Autodesk Inventor part; units mm, degrees
ref_plane "YZ Plane" through (0, 0, 0) normal (1, 0, 0) x (0, 1, 0)
ref_plane "XZ Plane" through (0, 0, 0) normal (0, 1, 0) x (-1, 0, 0)
ref_plane "XY Plane" through (0, 0, 0) normal (0, 0, 1) x (1, 0, 0)
sketch "Sketch1" plane through (0, 0, 0) normal (0, 1, 0) x (-1, 0, 0)
  line L0 (0, 0) -> (-457.2, 0)
  line L1 (-457.2, 0) -> (-457.2, -457.2)
  line L2 (-457.2, -457.2) -> (0, -457.2)
  line L3 (0, -457.2) -> (0, 0)
  dimension "d0" = 457.2
  dimension "d1" = 457.2
extrude "Extrusion1" add sketch "Sketch1" along normal blind 381
sketch "Sketch2" plane through (0, 381, 0) normal (0, 1, 0) x (1, 0, 0)
  line L0 (0, 0) -> (457.2, 0)
  line L1 (457.2, 0) -> (457.2, 457.2)
  line L2 (457.2, 457.2) -> (0, 457.2)
  line L3 (0, 457.2) -> (0, 0)
  line L4 (12.7, 12.7) -> (444.5, 12.7)
  line L5 (444.5, 12.7) -> (444.5, 444.5)
  line L6 (444.5, 444.5) -> (12.7, 444.5)
  line L7 (12.7, 444.5) -> (12.7, 12.7)
  dimension "d4" = 12.7
extrude "Extrusion2" cut sketch "Sketch2" against normal blind 368.3 contours L7 L6 L5 L4
sketch "Sketch3" plane through (0, 0, 0) normal (0, -1, 0) x (1, 0, 0)
  line L0 (0, 0) -> (457.2, 0)
  line L1 (0, -457.2) -> (0, 0)
  line L2 (457.2, -457.2) -> (0, -457.2)
  line L3 (457.2, 0) -> (457.2, -457.2)
  line L4 (457.2, 0) -> (406.4, 0) construction
  line L5 (0, 0) -> (457.2, 0) construction
  line L6 (406.4, 0) -> (406.4, -76.2) construction
  circle A0 centre (406.4, -76.2) radius 15.875
  line L7 (457.2, 0) -> (457.2, -457.2) construction
  line L8 (457.2, -228.6) -> (0, -228.6) construction
  line L9 (228.6, 0) -> (228.6, -457.2) construction
  circle A1 centre (406.4, -381) radius 15.875
  circle A2 centre (50.8, -381) radius 15.875
  circle A3 centre (50.8, -76.2) radius 15.875
  point P0 (228.6, -228.6)
  dimension "d7" = 50.8
  dimension "d8" = 76.2
  dimension "d9" = 31.75
extrude "Extrusion3" cut sketch "Sketch3" against normal blind 25.4 contours A0 | A1 | A2 | A3
sketch "Sketch5" plane through (0, 12.7, 0) normal (0, 1, 0) x (1, 0, 0)
  circle A0 centre (50.8, 381) radius 15.875
  circle A1 centre (406.4, 76.2) radius 15.875
  circle A2 centre (406.4, 381) radius 15.875
  circle A3 centre (50.8, 76.2) radius 15.875
  line L0 (444.5, 12.7) -> (12.7, 12.7)
  line L1 (444.5, 444.5) -> (444.5, 12.7)
  line L2 (12.7, 444.5) -> (444.5, 444.5)
  line L3 (12.7, 12.7) -> (12.7, 444.5)
  circle A4 centre (50.8, 381) radius 22.225
  circle A5 centre (406.4, 381) radius 22.225
  circle A6 centre (50.8, 76.2) radius 22.225
  circle A7 centre (406.4, 76.2) radius 22.225
  point P0 (0, 0)
  dimension "d19" = 6.35
  dimension "d20" = 6.35
  dimension "d21" = 6.35
  dimension "d22" = 6.35
extrude "Extrusion5" add sketch "Sketch5" along normal blind 12.7 contours A4 | A5 | A6 | A7
properties part number "Attachable top" material "PET Plastic"
CAD build for the part. Positions are in the model's coordinates, mm. A direction names the side the tool comes from. Coordinates: 2 decimals unless noted, no trailing zeros. Order: outer loops, then holes, each group sorted by start corner. A loop starts at its lowest first (then second) coordinate and runs counter-clockwise, first axis right, second up. Notation, with made-up numbers: M 53,-33.5 L 57,-33.5 A22 ccw 57,2.5 Z; hole C 33,58.25 d5. An arc over 180 degrees is marked long. Answer as CSV lines item,"result".
1) Cut at A-A (x = 50.8). List the corners of the cut face in (y, z) (3 decimals).
Verdict:
outline,"M 0,-457.2 L 381,-457.2 L 381,-444.5 L 12.7,-444.5 L 12.7,-403.225 L 25.4,-403.225 L 25.4,-396.875 L 0,-396.875 Z; M 0,-365.125 L 25.4,-365.125 L 25.4,-358.775 L 12.7,-358.775 L 12.7,-98.425 L 25.4,-98.425 L 25.4,-92.075 L 0,-92.075 Z; M 0,-60.325 L 25.4,-60.325 L 25.4,-53.975 L 12.7,-53.975 L 12.7,-12.7 L 381,-12.7 L 381,0 L 0,0 Z"
2) 3-axis set-ups, long thin cutter, end or side, ignore diameter. For faces 1 (the flat face through (457.2, 188, -225)), 2 (the flat face through (232, 199, -444.5)): which of +Z, -Z, +X, -X, +Y, -Y reach the whole face in a straight line?
Verdict:
face 1,"+Z, -Z, +X, +Y, -Y"
face 2,"+Y"
3) Flat gauge pins, fed straight in: P1, Ø13.5, axis at x = 395.5, z = -72, coming from the +Y side; P2, Ø19, axis at x = 50.8, z = -381, coming from the +Y side. Where does each tip first touch, or does it go through?
Verdict:
P1,"y = 25.4"
P2,"through"
4) Cut at C-C (z = -381). List the corners of the cut face in (x, y) (3 decimals), then the cut area to 3 significant figures.
Verdict:
outline,"M 0,0 L 34.925,0 L 34.925,25.4 L 28.575,25.4 L 28.575,12.7 L 12.7,12.7 L 12.7,381 L 0,381 Z; M 66.675,0 L 390.525,0 L 390.525,25.4 L 384.175,25.4 L 384.175,12.7 L 73.025,12.7 L 73.025,25.4 L 66.675,25.4 Z; M 422.275,0 L 457.2,0 L 457.2,381 L 444.5,381 L 444.5,12.7 L 428.625,12.7 L 428.625,25.4 L 422.275,25.4 Z"
area,"14,700 mm2"
5) Mould opens along X. For faces 3 (the flat face through (0, 188, -232)), 4 (the cylindrical face through (34.4, 19, -61.2)), 5 (the flat face through (232, 188, -457.2)) say: released by +X, released by -X, zero draft, split by the parting line, or undercut.
Verdict:
face 3,"released by -X"
face 4,"undercut"
face 5,"zero draft"
6) Drill centre lines: L1, parallel to X at y = 12.75, z = -76.2 (3 decimals); L2, parallel to Z at x = 50, y = 20; L3, parallel to X at y = 11, z = -76. Where is each one in solid material? Low to high. Write a range as from..to.
Verdict:
L1,"0..12.7, 28.575..34.925, 66.675..73.025, 384.175..390.525, 422.275..428.625, 444.5..457.2"
L2,"-457.2..-444.5, -403.21..-396.85, -365.15..-358.79, -98.41..-92.05, -60.35..-53.99, -12.7..0"
L3,"0..34.93, 66.67..390.53, 422.27..457.2"
7) Cut at D-D (x = 112.5). List the corners of the cut face in (y, z), then the cut area to 3 significant figures.
Verdict:
outline,"M 0,-457.2 L 381,-457.2 L 381,-444.5 L 12.7,-444.5 L 12.7,-12.7 L 381,-12.7 L 381,0 L 0,0 Z"
area,"15,200 mm2"
8) Cut at B-B (y = 138). List the corners of the cut face in (x, z), then the cut area to 3 significant figures.
Verdict:
outline,"M 0,-457.2 L 457.2,-457.2 L 457.2,0 L 0,0 Z; hole M 12.7,-444.5 L 444.5,-444.5 L 444.5,-12.7 L 12.7,-12.7 Z"
area,"22,600 mm2"
